Can you work these out from the model? Positions are in its coordinate system, mm. A direction names the side the tool comes from. Coordinates: 2 decimals unless noted, no trailing zeros. Order: outer loops, then holes, each group sorted by start corner. A loop starts at its lowest first (then second) coordinate and runs counter-clockwise, first axis right, second up. Notation, with made-up numbers: (48.5, 39.25) -> (89.5, 39.25) arc R22 ccw to (89.5, 70.25) -> close; hole circle Ø11 at (73, -29). An arc over 180 degrees is marked (long way). Use a Markdown table: item, result. Add a question column.
1. For faces 5 (the cylindrical face through (16.481, 8.022, 2.465)), 6 (the flat face through (34.75, 11, 2)), 7 (the cylindrical face through (13.4, -1.2, 2.5)), which set-ups out of +Z, -Z, +X, -X, +Y, -Y let a thin tool reach every point of the face, with its end or its side?
2. We'd pull the mould along Y, two halves only. Please class faces 1 (the cylindrical face through (30.92, 15.75, 2.46)), 2 (the cylindrical face through (-1.5, 0.07, 2.46)), 3 (the cylindrical face through (39.246, -3.606, 2.465)), 4 (the cylindrical face through (31.715, 8.725, 2.465)): pulls with the +Y half, pulls with the -Y half, needs draft (parallel to the pull), parting line crosses it, or undercut.
3. For pin 1 Ø1.5 at (y, z) = (2.5, 3.5) entering from +X; pin 2 Ø0.5 at (y, z) = (11, 2) entering from +X; pin 3 Ø3 at (x, y) = (15, 0) entering from -Z (1 decimal), each with a flat end and sliding along its axis, tell me the tip position at first contact or that it passes through.
4. Suppose I cut it at D-D, the plane z = 3.9. List the corners of the cut face in (x, y) for me.
5. If I drill on line 1 along Y through (x, z) = (31, 2.15); line 2 along X through (y, z) = (-1, 3.15); line 3 along Y through (x, z) = (6, 2.5), over which ranges is the centre line in solid material (lowest first)? Write a range as from..to.
6. Suppose I cut it at A-A, the plane x = 31. List the corners of the cut face in (y, z) for me.
7. Suppose I cut it at B-B, the plane y = 0. List the corners of the cut face in (x, z) for me, then the cut area to 3 significant figures.
8. Suppose I cut it at C-C, the plane x = 0. List the corners of the cut face in (y, z) for me, then the cut area to 3 significant figures.
```python
from build123d import *

# Parameters (mm, degrees)
SKETCH1_R           = 1.5
SKETCH1_R_2         = 1.25
SKETCH1_R_3         = 2
SKETCH1_R_4         = 1
SKETCH1_R_5         = 0.75
BOSS_EXTRUDE1_DEPTH = 5


with BuildPart() as part:
    # Sketch1 → Boss-Extrude1 (new body)
    with BuildSketch(Plane.XY):
        with BuildLine():
            Line((18.457499004, 7.5), (23.25, 7.5))
            ThreePointArc((23.25, 7.5), (26.078427125, 8.671572875), (27.25, 11.5))
            Line((27.25, 11.5), (27.25, 12))
            ThreePointArc((27.25, 12), (31, 15.75), (34.75, 12))
            Line((34.75, 12), (34.75, 10.437312873))
            ThreePointArc((34.75, 10.437312873), (35.176593954, 8.639878804), (36.365384615, 7.225831989))
            ThreePointArc((36.365384615, 7.225831989), (39.175605476, -3.762907798), (29.000770207, -8.775139898))
            ThreePointArc((29.000770207, -8.775139898), (15.040769607, -6.867204956), (0.962557604, -7.437975723))
            ThreePointArc((0.962557604, -7.437975723), (-3.385742672, -6.692290083), (-6.5625, -3.630921887))
            ThreePointArc((-6.5625, -3.630921887), (-7.966305911, 3.694931991), (-4.770712178, 10.434886499))
            Line((-4.770712178, 10.434886499), (-3.879663294, 11.374703534))
            ThreePointArc((-3.879663294, 11.374703534), (6.070726491, 15.053905129), (15.050261475, 9.404592542))
            ThreePointArc((15.050261475, 9.404592542), (16.505785633, 8.008465249), (18.457499004, 7.5))
        make_face()
        Circle(SKETCH1_R, mode=Mode.SUBTRACT)
        with Locations((31, 0)):
            Circle(SKETCH1_R_2, mode=Mode.SUBTRACT)
        with Locations((15, 0)):
            Circle(SKETCH1_R_3, mode=Mode.SUBTRACT)
        with Locations((6, 13)):
            Circle(SKETCH1_R_4, mode=Mode.SUBTRACT)
        with Locations((31, 8.5)):
            Circle(SKETCH1_R_5, mode=Mode.SUBTRACT)
    extrude(amount=BOSS_EXTRUDE1_DEPTH)


solid = part.part
```
Worked out:
| question | item | result |
|---|---|---|
| 1 | face 5 | +Z, -Z, +Y |
| 1 | face 6 | +Z, -Z, +X, +Y |
| 1 | face 7 | +Z, -Z |
| 2 | face 1 | pulls with the +Y half |
| 2 | face 2 | undercut |
| 2 | face 3 | parting line crosses it |
| 2 | face 4 | undercut |
| 3 | pin 1 | stops at x = 39.83 |
| 3 | pin 2 | stops at x = 34.75 |
| 3 | pin 3 | passes through |
| 4 | outline | (-6.56, -3.63) arc R7.5 ccw to (0.96, -7.44) arc R80 cw to (29, -8.78) arc R9 ccw to (36.37, 7.23) arc R4 cw to (34.75, 10.44) -> (34.75, 12) arc R3.75 ccw to (27.25, 12) -> (27.25, 11.5) arc R4 cw to (23.25, 7.5) -> (18.46, 7.5) arc R4 cw to (15.05, 9.4) arc R12 ccw to (-3.88, 11.37) -> (-4.77, 10.43) arc R12 ccw to start; hole circle Ø3 at (0, 0); hole circle Ø2 at (6, 13); hole circle Ø4 at (15, 0); hole circle Ø2.5 at (31, 0); hole circle Ø1.5 at (31, 8.5) |
| 5 | line 1 | y = -9..-1.25, 1.25..7.75, 9.25..15.75 |
| 5 | line 2 | x = -7.63..-1.12, 1.12..13.27, 16.73..30.25, 31.75..39.94 |
| 5 | line 3 | y = -6.95..12, 14..15.06 |
| 6 | outline | (-9, 0) -> (-1.25, 0) -> (-1.25, 5) -> (-9, 5) -> close; (1.25, 0) -> (7.75, 0) -> (7.75, 5) -> (1.25, 5) -> close; (9.25, 0) -> (15.75, 0) -> (15.75, 5) -> (9.25, 5) -> close |
| 7 | outline | (-7.86, 0) -> (-1.5, 0) -> (-1.5, 5) -> (-7.86, 5) -> close; (1.5, 0) -> (13, 0) -> (13, 5) -> (1.5, 5) -> close; (17, 0) -> (29.75, 0) -> (29.75, 5) -> (17, 5) -> close; (32.25, 0) -> (40, 0) -> (40, 5) -> (32.25, 5) -> close |
| 7 | area | 192 mm² |
| 8 | outline | (-7.5, 0) -> (-1.5, 0) -> (-1.5, 5) -> (-7.5, 5) -> close; (1.5, 0) -> (14.1, 0) -> (14.1, 5) -> (1.5, 5) -> close |
| 8 | area | 93.0 mm² |
